Geometry: see drawing. Coordinates: mm, zero at the bounding-box minimum. A direction names the side the tool comes from. Give positions to 0.01 mm unless a question says otherwise; leave off trailing zeros. Loops run counter-clockwise (first coordinate to the right, second up) from the corner with the lowest first, then second, coordinate; pieces in that order, holes last. Notation, with made-up numbers: M -24,61.25 L 11,61.25 A20 ccw 11,83.25 Z; hole C 81,61 d8. An arc over 180 degrees is marked long. Put each result on its own line as item: value.
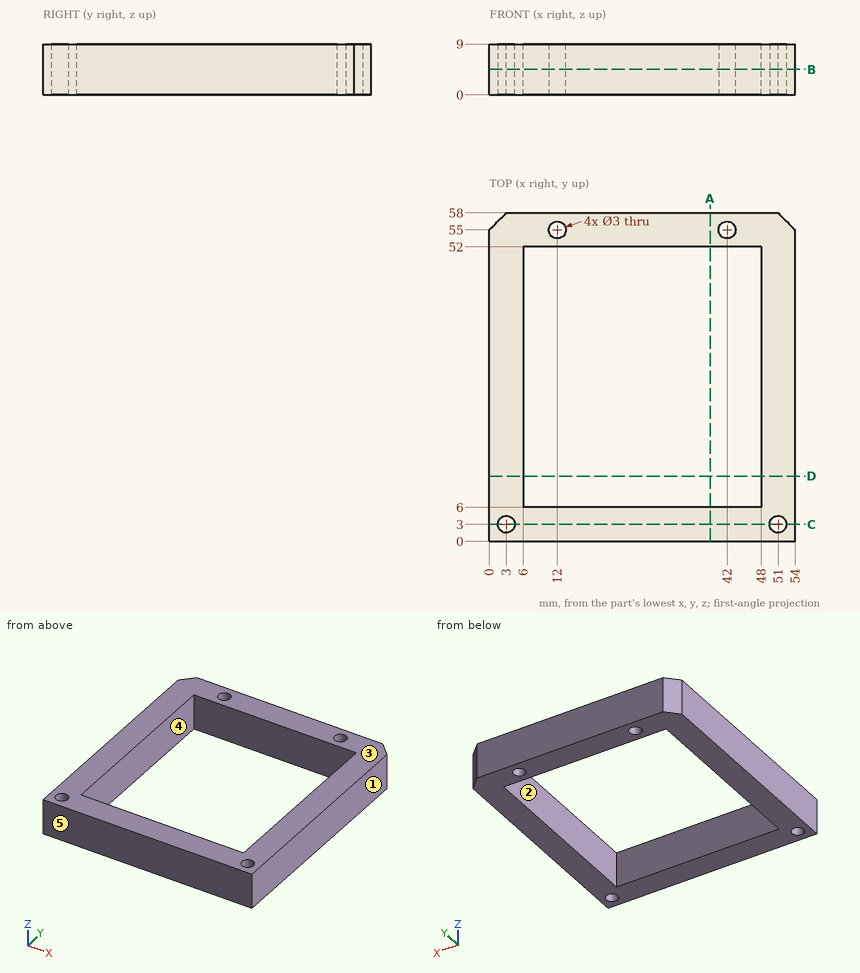
Item 1: Set-up query: the marked faces 1 and 2. Return all of +Z, -Z, +X, -X, +Y, -Y with unobstructed straight access to the full face (end or side cutting, diameter ignored); none if empty.
Output values:
face 1: +Z, -Z, +X, +Y, -Y
face 2: +Z, -Z
Item 2: Section C-C on y = 3. Output: boundary loops of the cut face in (x, z).
Output values:
outline: M 0,0 L 1.5,0 L 1.5,9 L 0,9 Z; M 4.5,0 L 49.5,0 L 49.5,9 L 4.5,9 Z; M 52.5,0 L 54,0 L 54,9 L 52.5,9 Z
Item 3: Mould query, pull axis Y, two halves, no side actions, for the marked faces 3, 4 and 5. Classes: pulls with the +Y half, pulls with the -Y half, needs draft (parallel to the pull), parting line crosses it, or undercut.
Output values:
face 3: needs draft
face 4: undercut
face 5: pulls with the -Y half
Item 4: Line query: probe 1 along Y at (x, z) = (42, 7); probe 2 along X at (y, z) = (3, 7); probe 3 along X at (y, z) = (48, 7.75). Output: solid intervals per line, ascending. Write a range as [from, to].
Output values:
probe 1: [0, 6], [52, 53.5], [56.5, 58]
probe 2: [0, 1.5], [4.5, 49.5], [52.5, 54]
probe 3: [0, 6], [48, 54]
Item 5: Section A-A on x = 39. Output: boundary loops of the cut face in (y, z).
Output values:
outline: M 0,0 L 6,0 L 6,9 L 0,9 Z; M 52,0 L 58,0 L 58,9 L 52,9 Z
Item 6: Section B-B on z = 4.5. Output: boundary loops of the cut face in (x, y), then the cut area to 3 significant figures.
Output values:
outline: M 0,0 L 54,0 L 54,55 L 51,58 L 3,58 L 0,55 Z; hole C 3,3 d3; hole M 6,6 L 48,6 L 48,52 L 6,52 Z; hole C 12,55 d3; hole C 42,55 d3; hole C 51,3 d3
area: 1,160 mm²
Item 7: Section D-D on y = 11.5. Output: boundary loops of the cut face in (x, z).
Output values:
outline: M 0,0 L 6,0 L 6,9 L 0,9 Z; M 48,0 L 54,0 L 54,9 L 48,9 Z
